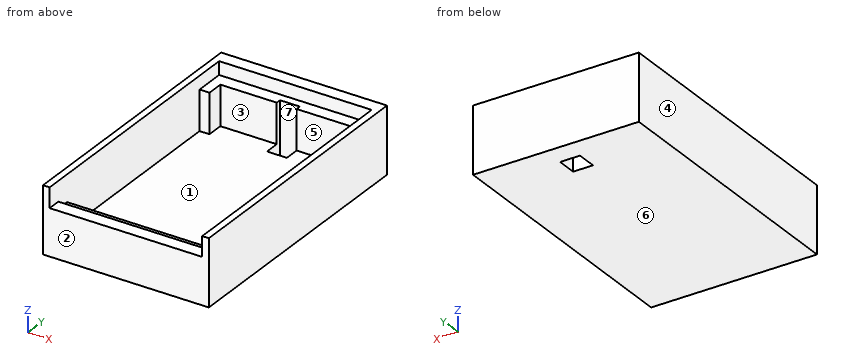
from build123d import *

# Parameters (mm, degrees)
SKETCH_W        = 25
SKETCH_H        = 41
PAD_DEPTH       = 10
SKETCH001_W     = 23
SKETCH001_H     = 37
POCKET_DEPTH    = 2
SKETCH002_W     = 23
SKETCH002_H     = 33
POCKET001_DEPTH = 6
SKETCH003_W     = 23
SKETCH003_H     = 2
POCKET002_DEPTH = 4
SKETCH005_W     = 23
SKETCH005_H     = 6
POCKET003_DEPTH = 3
SKETCH006_W     = 3
SKETCH006_H     = 3
POCKET004_DEPTH = 8.001
SKETCH012_W     = 1.5
SKETCH012_H     = 2.5
PAD004_DEPTH    = 6


with BuildPart() as part:
    # Sketch → Pad (new body)
    with BuildSketch(Plane.XY):
        Rectangle(SKETCH_W, SKETCH_H)
    extrude(amount=PAD_DEPTH)

    # Sketch001 (on Face6 of Pad) → Pocket (cut)
    with BuildSketch(Plane.XY.offset(10)):
        Rectangle(SKETCH001_W, SKETCH001_H)
    extrude(amount=-POCKET_DEPTH, mode=Mode.SUBTRACT)

    # Sketch002 (on Face11 of Pocket) → Pocket001 (cut)
    with BuildSketch(Plane.XY.offset(8)):
        Rectangle(SKETCH002_W, SKETCH002_H)
    extrude(amount=-POCKET001_DEPTH, mode=Mode.SUBTRACT)

    # Sketch003 (on Face5 of Pocket001) → Pocket002 (cut)
    with BuildSketch(Plane.XY.offset(10)):
        with Locations((0, -17.5)):
            Rectangle(SKETCH003_W, SKETCH003_H)
    extrude(amount=-POCKET002_DEPTH, mode=Mode.SUBTRACT)

    # Sketch005 (on Face5 of Pocket002) → Pocket003 (cut)
    with BuildSketch(Plane.XY.offset(10)):
        with Locations((0, -19.5)):
            Rectangle(SKETCH005_W, SKETCH005_H)
    extrude(amount=-POCKET003_DEPTH, mode=Mode.SUBTRACT)

    # Sketch006 (on Face16 of Pocket003) → Pocket004 (cut, through all)
    with BuildSketch(Plane.XY.offset(8)):
        with Locations((0, 15.75)):
            Rectangle(SKETCH006_W, SKETCH006_H)
    extrude(amount=-POCKET004_DEPTH, mode=Mode.SUBTRACT)

    # Sketch012 (on Face21 of Pocket004) → Pad004 (join)
    with BuildSketch(Plane.XY.offset(2)):
        with Locations((-10.75, 15.25)):
            Rectangle(SKETCH012_W, SKETCH012_H)
        with Locations((10.75, 15.25)):
            Rectangle(SKETCH012_W, SKETCH012_H)
    extrude(amount=PAD004_DEPTH)


solid = part.part
Geometry: final body of the model. Coordinates: model frame, mm. Face numbers are marked on the shaded views. A direction names the side the tool comes from. Give positions to 0.01 mm unless a question says otherwise; leave off trailing zeros. Loops run counter-clockwise (first coordinate to the right, second up) from the corner with the lowest first, then second, coordinate; pieces in that order, holes last. Notation, with made-up numbers: (78, 54.5) - (130, 54.5) arc R26 ccw to (130, 89.5) - close; hole circle Ø3 at (52, 82.25). An arc over 180 degrees is marked (long way). Answer as CSV lines item,"result". Start each with the question number.
1. Ray query, L1, parallel to Y at x = 5, z = 2.25; L2, parallel to X at y = -14, z = 4.75; L3, parallel to Y at x = -11, z = 3. Return the intervals inside material, ascending.
2. Section A-A, the plane x = 1. Return loops of the section in (y, z), plus the area to 4 significant figures.
3. Section C-C, the plane y = 18. Return loops of the section in (x, z).
4. Section D-D, the plane x = 6.5. Return loops of the section in (y, z), plus the area to 3 significant figures.
5. Draft query along Y for the marked faces 1, 2, 3 and 4. Return one class per face: released by +Y, released by -Y, zero draft, split by the parting line, or undercut.
6. Reachability of the marked faces 5, 6 and 7 from +Z, -Z, +X, -X, +Y, -Y: full face, straight path, thin tool, end or side. Return the list, or none.
7. Section B-B, the plane z = 3. Return loops of the section in (x, y), plus the area to 3 significant figures.
8. Pin query (flat end, axial travel): P1, Ø12, axis at x = -3.5, y = 6, coming from the +Z side; P2, Ø0.6, axis at x = -3.5, y = -17.5, coming from the +Z side. Return the tip coordinate at first contact, or that it passes through.
Answers:
1,L1,"y = -20.5 to -16.5, 16.5 to 20.5"
1,L2,"x = -12.5 to -11.5, 11.5 to 12.5"
1,L3,"y = -20.5 to -16.5, 14 to 20.5"
2,outline,"(-20.5, 0) - (14.25, 0) - (14.25, 2) - (-16.5, 2) - (-16.5, 6) - (-18.5, 6) - (-18.5, 7) - (-20.5, 7) - close; (17.25, 0) - (20.5, 0) - (20.5, 10) - (18.5, 10) - (18.5, 8) - (17.25, 8) - close"
2,area,"117.5 mm2"
3,outline,"(-12.5, 0) - (12.5, 0) - (12.5, 10) - (11.5, 10) - (11.5, 8) - (-11.5, 8) - (-11.5, 10) - (-12.5, 10) - close"
4,outline,"(-20.5, 0) - (20.5, 0) - (20.5, 10) - (18.5, 10) - (18.5, 8) - (16.5, 8) - (16.5, 2) - (-16.5, 2) - (-16.5, 6) - (-18.5, 6) - (-18.5, 7) - (-20.5, 7) - close"
4,area,"128 mm2"
5,face 1,"undercut"
5,face 2,"released by -Y"
5,face 3,"undercut"
5,face 4,"zero draft"
6,face 5,"+Z"
6,face 6,"-Z, +X, -X, +Y, -Y"
6,face 7,"+Z, -Z"
7,outline,"(-12.5, -20.5) - (12.5, -20.5) - (12.5, 20.5) - (-12.5, 20.5) - close; hole (-11.5, -16.5) - (11.5, -16.5) - (11.5, 14) - (10, 14) - (10, 16.5) - (1.5, 16.5) - (1.5, 17.25) - (-1.5, 17.25) - (-1.5, 16.5) - (-10, 16.5) - (-10, 14) - (-11.5, 14) - close"
7,area,"271 mm2"
8,P1,"stops at z = 2"
8,P2,"stops at z = 6"
